```python
from build123d import *

# Parameters (mm, degrees)
F1_DEPTH = 76.2
F3_DEPTH = 152.4


with BuildPart() as f1:
    # F0 (on Front) → F1 (new body)
    with BuildSketch(Plane.XZ):
        Polygon((0, 50.8), (0, 0), (152.4, 0), (152.4, 38.1), (116.141342, 38.1), (107.95, 50.8), (82.55, 50.8), (82.55, 38.1), (95.25, 38.1), (95.25, 25.4), (82.55, 25.4), (12.7, 25.4), (12.7, 38.1), (25.4, 38.1), (25.4, 50.8), align=None)
    extrude(amount=F1_DEPTH)

    # F2 (on face) → F3 (cut)
    with BuildSketch(Plane.YZ.offset(152.4)):
        Polygon((-12.7, 12.7), (-38.1, 12.7), (-63.5, 12.7), (-50.8, 0), (-25.4, 0), align=None)
    extrude(amount=-F3_DEPTH, mode=Mode.SUBTRACT)


solid = f1.part
```
Geometry: final body of the model. Coordinates: model frame, mm. A direction names the side the tool comes from. Coordinates: 2 decimals unless noted, no trailing zeros. Loops run counter-clockwise (first coordinate to the right, second up) from the corner with the lowest first, then second, coordinate; pieces in that order, holes last. Notation, with made-up numbers: M -18.75,51.5 L 20.25,51.5 A11 cw 20.25,71.5 Z; hole C -18.5,11 d8. An arc over 180 degrees is marked long. Put each result on its own line as item: value.
(1) Material intervals for probe 1 along X at (y, z) = (-64, 37); probe 2 along Z at (x, y) = (89.5, -35.5); probe 3 along Z at (x, y) = (25, -65.5), sorted ascending.
Answer sheet:
probe 1: x = 0 to 12.7, 95.25 to 152.4
probe 2: z = 12.7 to 25.4, 38.1 to 50.8
probe 3: z = 0 to 25.4, 38.1 to 50.8
(2) Draft query along Y for faces 1 (the face through (77.3, -19.1, 6.3)), 2 (the face through (75, 0, 20)), 3 (the face through (75, -63, 0)). Return one class per face: pulls with the +Y half, pulls with the -Y half, needs draft (parallel to the pull), parting line crosses it, or undercut.
Answer sheet:
face 1: undercut
face 2: pulls with the +Y half
face 3: needs draft
(3) Cut plane D-D on x = 35. Return the cut outline in (y, z).
Answer sheet:
outline: M -76.2,0 L -50.8,0 L -63.5,12.7 L -12.7,12.7 L -25.4,0 L 0,0 L 0,25.4 L -76.2,25.4 Z
(4) First-contact query: pin 1 (6.5 mm diameter, centred on x = 89.5, y = -35.5, fed in from -Z); pin 2 (1 mm diameter, centred on x = 67, y = -45, fed in from +Z); pin 3 (18 mm diameter, centred on x = 141, y = -56.5, fed in from +Z). Flat tips, straight axial feed; report the tip coordinate or a pass-through.
Answer sheet:
pin 1: stops at z = 12.7
pin 2: stops at z = 25.4
pin 3: stops at z = 38.1
(5) Cut plane C-C on x = 86.5. Return the cut outline in (y, z), then the cut area to 3 significant figures.
Answer sheet:
outline: M -76.2,0 L -50.8,0 L -63.5,12.7 L -12.7,12.7 L -25.4,0 L 0,0 L 0,25.4 L -76.2,25.4 Z; M -76.2,38.1 L 0,38.1 L 0,50.8 L -76.2,50.8 Z
area: 2,420 mm^2
(6) Cut plane B-B on z = 9.5. Return the cut outline in (x, y).
Answer sheet:
outline: M 0,-76.2 L 152.4,-76.2 L 152.4,-60.3 L 0,-60.3 Z; M 0,-15.9 L 152.4,-15.9 L 152.4,0 L 0,0 Z
(7) Access query for faces 4 (the face through (89, -38, 38.1)), 5 (the face through (82.55, -38, 45)), 6 (the face through (135, -38, 38.1)). Directions: +Z, -Z, +X, -X, +Y, -Y. A direction counts if a zero-diameter tool reaches every point of the face in a straight line with its end or side. Return the directions, or none.
Answer sheet:
face 4: +Y, -Y
face 5: +Z, +Y, -Y
face 6: +Z, +X, +Y, -Y
(8) Cut plane A-A on y = -17. Return the cut outline in (x, z), then the cut area to 3 significant figures.
Answer sheet:
outline: M 0,0 L 152.4,0 L 152.4,8.4 L 0,8.4 Z; M 0,12.7 L 152.4,12.7 L 152.4,38.1 L 116.14,38.1 L 107.95,50.8 L 82.55,50.8 L 82.55,38.1 L 95.25,38.1 L 95.25,25.4 L 12.7,25.4 L 12.7,38.1 L 25.4,38.1 L 25.4,50.8 L 0,50.8 Z
area: 4,800 mm^2
